Source: CAD feature listing. Evaluate the final solid. Frame: model axes, mm. Give positions to 0.01 mm unless a question says otherwise; leave off trailing zeros. Order: outer loops, then holes, each group sorted by start corner. A loop starts at its lowest first (then second) coordinate and runs counter-clockwise, first axis right, second up. Notation, with made-up numbers: M 66.25,44 L 91.25,44 A19 ccw 91.25,72 Z; hole C 38.25,-30 d2. An arc over 180 degrees is marked long. Use CSV: the item, a comma, the result in double quotes. Start each with the question number.
Item 1: Section query C-C on x = 0.5. Return loops of the section in (y, z).
Item 2: Ray query, probe 1 along X at (y, z) = (1.4, -25); probe 2 along X at (y, z) = (0.55, 29). Return the intervals inside material, ascending. Write a range as from..to.
Item 3: First-contact query: pin 1 (1 mm diameter, centred on x = -0.5, y = 1.5, fed in from +Z). Flat tip, straight axial feed; report the tip coordinate or a pass-through.
Item 4: Section query A-A on x = 30. Return loops of the section in (y, z).
Item 5: Section query B-B on z = 26.5. Return loops of the section in (x, y), and give its area (3 significant figures).
from build123d import *

# Parameters (mm, degrees)
SKETCH1_W           = 82
SKETCH1_H           = 82
BOSS_EXTRUDE1_DEPTH = 2
CUT_EXTRUDE2_DEPTH  = 10


with BuildPart() as part:
    # Sketch1 → Boss-Extrude1 (new body)
    with BuildSketch(Plane(origin=(0, 0, 0), x_dir=(1, 0, 0), z_dir=(0, 1, 0))):
        Rectangle(SKETCH1_W, SKETCH1_H)
    extrude(amount=BOSS_EXTRUDE1_DEPTH)

    # Sketch2 → Cut-Extrude2 (cut)
    with BuildSketch(Plane(origin=(0, 0, 0), x_dir=(-1, 0, 0), z_dir=(0, -1, 0))):
        Polygon((-1.5, 22.5), (1.5, 22.5), (1.5, 28.3), (4, 28.3), (4, 31.75), (1.5, 31.75), (1.5, 41), (-1.5, 41), (-1.5, 31.75), (-4, 31.75), (-4, 28.3), (-1.5, 28.3), align=None)
        Polygon((28.3, -4), (28.3, -1.5), (22.5, -1.5), (22.5, 1.5), (28.3, 1.5), (28.3, 4), (31.75, 4), (31.75, 1.5), (41, 1.5), (41, -1.5), (31.75, -1.5), (31.75, -4), align=None)
        Polygon((-4, -28.3), (-1.5, -28.3), (-1.5, -22.5), (1.5, -22.5), (1.5, -28.3), (4, -28.3), (4, -31.75), (1.5, -31.75), (1.5, -41), (-1.5, -41), (-1.5, -31.75), (-4, -31.75), align=None)
        Polygon((-28.3, 4), (-28.3, 1.5), (-22.5, 1.5), (-22.5, -1.5), (-28.3, -1.5), (-28.3, -4), (-31.75, -4), (-31.75, -1.5), (-41, -1.5), (-41, 1.5), (-31.75, 1.5), (-31.75, 4), align=None)
    extrude(amount=-CUT_EXTRUDE2_DEPTH, mode=Mode.SUBTRACT)


solid = part.part
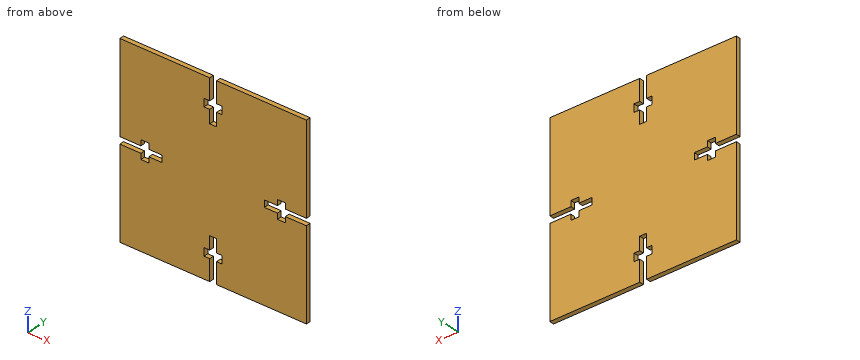
Verdict:
1,outline,"M 0,-22.5 L 2,-22.5 L 2,22.5 L 0,22.5 Z"
2,probe 1,"-41..-1.5, 1.5..41"
2,probe 2,"-41..-4, 4..41"
3,pin 1,"z = 22.5"
4,outline,"M 0,-41 L 2,-41 L 2,-4 L 0,-4 Z; M 0,4 L 2,4 L 2,41 L 0,41 Z"
5,outline,"M -41,0 L -1.5,0 L -1.5,2 L -41,2 Z; M 1.5,0 L 41,0 L 41,2 L 1.5,2 Z"
5,area,"158 mm2"
